Source: CAD feature listing. Evaluate the final solid. Frame: model axes, mm. Face numbers are marked on the shaded views. A direction names the side the tool comes from. Coordinates: 2 decimals unless noted, no trailing zeros. Write each loop counter-clockwise with the first axis right and the second up, starting at its lowest first coordinate (ties: lowest second). Pieces come first, ordered by that corner, then holes. Notation, with made-up numbers: (-24.5, -9.5) -> (25.5, -9.5) arc R16 cw to (25.5, -5.5) -> close; hole circle Ø2 at (-13, 44.5). An arc over 180 degrees is marked (long way). Write item = value, one per line.
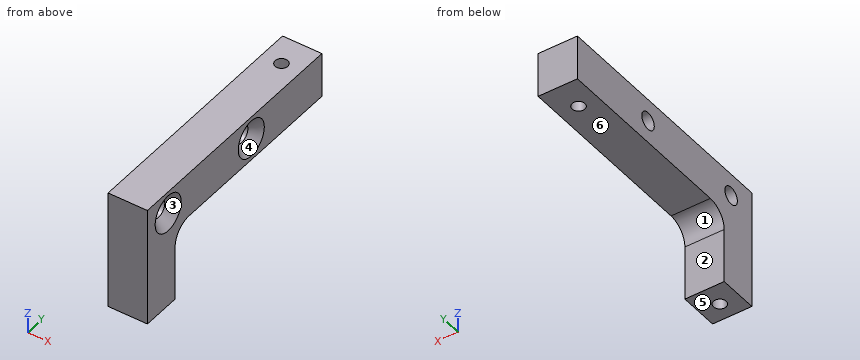
Autodesk Inventor part; units mm, degrees
ref_plane "YZ Plane" through (0, 0, 0) normal (1, 0, 0) x (0, 1, 0)
ref_plane "XZ Plane" through (0, 0, 0) normal (0, 1, 0) x (-1, 0, 0)
ref_plane "XY Plane" through (0, 0, 0) normal (0, 0, 1) x (1, 0, 0)
sketch "Sketch1" plane through (0, 0, 0) normal (0, 0, 1) x (1, 0, 0)
  line L0 (0, 0) -> (10, 0)
  line L1 (10, 0) -> (10, 63)
  line L2 (10, 63) -> (0, 63)
  line L3 (0, 63) -> (0, 0)
  dimension "d0" = 10
  dimension "d1" = 63
extrude "Extrusion1" add sketch "Sketch1" along normal blind 11.5
sketch "Sketch2" plane through (0, 0, 11.5) normal (0, 0, 1) x (1, 0, 0)
  line L0 (10, 63) -> (0, 63)
  line L1 (0, 0) -> (10, 0)
  point P0 (5, 55.5)
  point P1 (5, 63)
  dimension "d5" = 7.5
  dimension "d24" = 63
hole "Hole1" at (5, 55.5, 11.5) direction (0, 0, -1) diameter 3.242 end through all
sketch "Sketch3" plane through (10, 0, 0) normal (1, 0, 0) x (0, 0, -1)
  line L0 (0, 63) -> (-11.5, 63)
  line L1 (0, 0) -> (-11.5, 0)
  point P0 (-5.75, 37.5)
  point P1 (-5.75, 7.5)
  point P2 (-5.75, 63)
  dimension "d16" = 7.5
  dimension "d25" = 30
hole "Hole2" at (10, 37.5, 5.75) at (10, 7.5, 5.75) direction (-1, 0, 0) diameter 4.5 end through all countersink diameter 9.4 countersink angle 90
sketch "Sketch4" plane through (0, 0, 0) normal (0, 0, -1) x (-1, 0, 0)
  point P0 (0, 0)
sketch "Sketch5" plane through (0, 0, 0) normal (0, 0, -1) x (-1, 0, 0)
  line L0 (0, 0) -> (-10, 0)
  line L1 (-10, 0) -> (-10, 10)
  line L2 (-10, 10) -> (0, 10)
  line L3 (0, 10) -> (0, 0)
  line L4 (-10, 0) -> (-10, 63)
  dimension "d26" = 10
extrude "Extrusion2" add sketch "Sketch5" along normal blind 19
sketch "Sketch6" plane through (0, 0, -19) normal (0, 0, -1) x (-1, 0, 0)
  line L0 (-10, 0) -> (0, 0)
  line L1 (0, 10) -> (-10, 10)
  circle A0 centre (-5, 55.5) radius 1.621
  point P0 (-5, 4.5)
  point P1 (-5, 0)
  dimension "d31" = 51
hole "Hole3" at (5, 4.5, -19) direction (0, 0, 1) diameter 3.242 depth 11.8 tip angle 118
fillet "Fillet1" radius 5 1 edges at (5, 10, 0)
properties part number "Pancake_Flexi Pipe Mount 2" material "Aluminum 6061"
1) First-contact query: pin 1 Ø6 at (x, y) = (4.5, 37) entering from -Z; pin 2 Ø8 at (y, z) = (54, -7) entering from -X; pin 3 Ø5 at (x, z) = (3.5, -10.5) entering from +Y; pin 4 Ø1.5 at (x, y) = (8, 11.5) entering from -Z. Flat tips, straight axial feed; report the tip coordinate or a pass-through.
Answer block:
pin_1 = 0
pin_2 = through
pin_3 = 10
pin_4 = -2.37
2) Cut plane D-D, the plane z = 6.5. Give the number of separate pieces and of enclosed holes in the cut face, and give its area (3 significant figures).
Answer block:
separate_pieces = 3
enclosed_holes = 1
area = 524 mm2
3) Cut plane A-A, the plane y = 7.5. Output: boundary loops of the cut face in (x, z), and give its area (3 significant figures).
Answer block:
outline = (0, -19) -> (10, -19) -> (10, 1.05) -> (7.55, 3.5) -> (0, 3.5) -> close; (0, 8) -> (7.55, 8) -> (10, 10.45) -> (10, 11.5) -> (0, 11.5) -> close
area = 254 mm2
4) Cut plane C-C, the plane y = 37.5. Output: boundary loops of the cut face in (x, z), and give its area (3 significant figures).
Answer block:
outline = (0, 0) -> (10, 0) -> (10, 1.05) -> (7.55, 3.5) -> (0, 3.5) -> close; (0, 8) -> (7.55, 8) -> (10, 10.45) -> (10, 11.5) -> (0, 11.5) -> close
area = 64.0 mm2
5) Cut plane B-B, the plane x = 1.5. Output: boundary loops of the cut face in (y, z), and give its area (3 significant figures).
Answer block:
outline = (0, -19) -> (10, -19) -> (10, -5) arc R5 cw to (15, 0) -> (63, 0) -> (63, 11.5) -> (0, 11.5) -> close; hole circle Ø4.5 at (7.5, 5.75); hole circle Ø4.5 at (37.5, 5.75)
area = 888 mm2
6) Reachability of the marked faces 5 and 6 from +Z, -Z, +X, -X, +Y, -Y: full face, straight path, thin tool, end or side. Return the list, or none.
Answer block:
face_5 = -Z, +X, -X, +Y, -Y
face_6 = -Z, +X, -X, +Y
7) Pull-direction query (Z, two-part tool) for the marked faces 1, 2, 3 and 4; classes: +Z half, -Z half, draft (parallel to the pull), parting line (faces both ways), or undercut.
Answer block:
face_1 = -Z half
face_2 = draft
face_3 = undercut
face_4 = undercut
8) Material intervals for probe 1 along Y at (x, z) = (3, 5.75); probe 2 along Y at (x, z) = (5, -13.5); probe 3 along Z at (x, y) = (1.75, 37.5), sorted ascending. Write a range as [from, to].
Answer block:
probe_1 = [0, 5.25], [9.75, 35.25], [39.75, 63]
probe_2 = [0, 2.88], [6.12, 10]
probe_3 = [0, 3.5], [8, 11.5]
